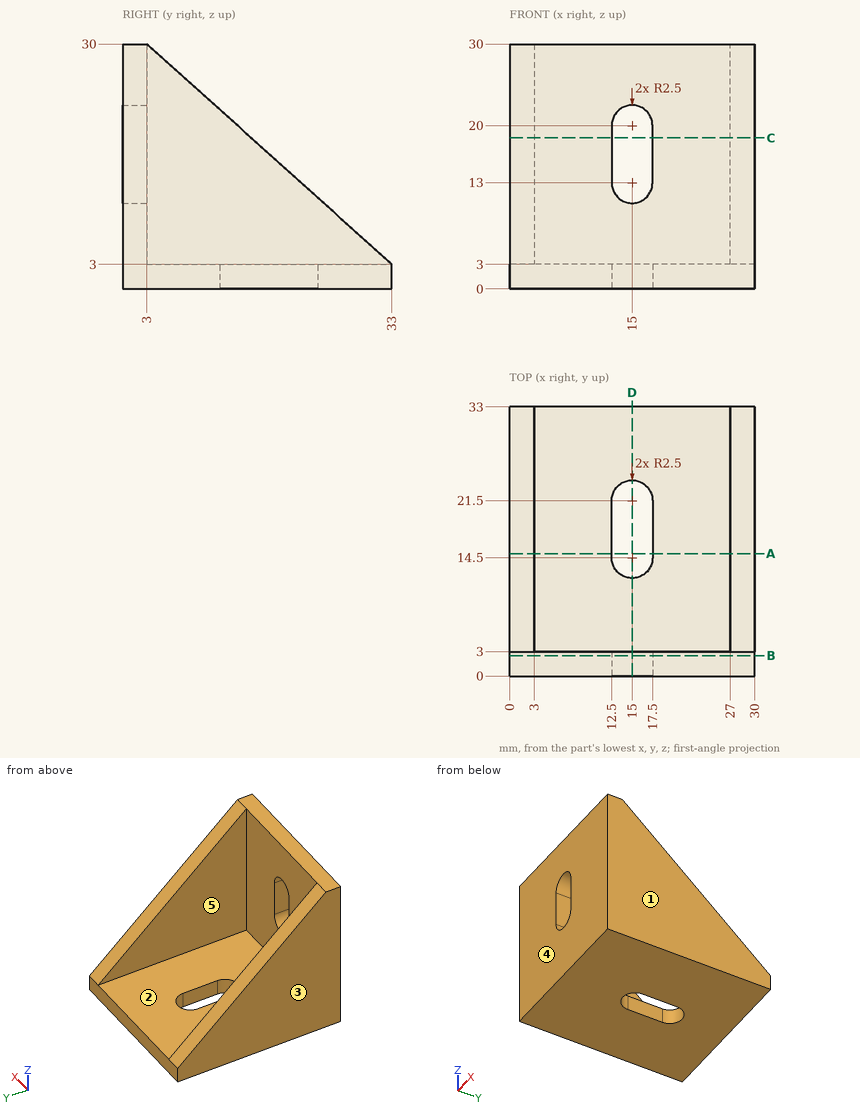
Answer from the drawing. Dimensions are ordinates in mm from the lowest x, y and z of the part. A direction names the side the tool comes from. Coordinates: 2 decimals unless noted, no trailing zeros. Write each loop counter-clockwise with the first axis right and the second up, starting at its lowest first coordinate (ties: lowest second). Pieces come first, ordered by that corner, then holes. Notation, with made-up numbers: (23.5, 44.25) - (58.5, 44.25) arc R17 ccw to (58.5, 75.25) - close; hole circle Ø2 at (72, -26.75). An arc over 180 degrees is marked (long way). Return JSON: item names as keys, results as strings. Group by question number.
Q1. The part is cut by section C-C on z = 18.5. Write down the section's boundary in (x, y).
Q2. The part is cut by section B-B on y = 2.5. Write down the section's boundary in (x, z), and give its area (3 significant figures).
Q3. The part is cut by section D-D on x = 15. Write down the section's boundary in (y, z).
Q4. Flat-ended cylindrical pins translate along their axes: pin 1 Ø1.5 at (x, y) = (22, 9.5) entering from +Z; pin 2 Ø8 at (x, z) = (8, 17.5) entering from +Y; pin 3 Ø6 at (x, y) = (25, 24) entering from +Z. Find the tip coordinate at first contact, or state that the pin passes through.
Q5. The part is cut by section A-A on y = 15. Write down the section's boundary in (x, z), and give its area (3 significant figures).
Q6. For a pull along X with two mould halves and no side action, classify the marked faces 3, 4 and 5 as +X half, -X half, draft (parallel to the pull), parting line (faces both ways), or undercut.
Q7. Which of the six approach directions +Z, -Z, +X, -X, +Y, -Y give full straight-line access (tool end or side, diameter ignored) to the marked faces 1 and 2?
Q8. Find the intervals of material crossed by line 1 along X through (y, z) = (12, 21.75); line 2 along X through (y, z) = (14.5, 1.25); line 3 along Y through (x, z) = (4, 23.25), in increasing order. Write a range as [from, to].
Evaluation:
{
 "1": {"outline": "(0, 0) - (12.5, 0) - (12.5, 3) - (3, 3) - (3, 15.78) - (0, 15.78) - close; (17.5, 0) - (30, 0) - (30, 15.78) - (27, 15.78) - (27, 3) - (17.5, 3) - close"},
 "2": {"outline": "(0, 0) - (30, 0) - (30, 30) - (0, 30) - close; hole (12.5, 13) arc R2.5 ccw to (17.5, 13) - (17.5, 20) arc R2.5 ccw to (12.5, 20) - close", "area": "845 mm2"},
 "3": {"outline": "(0, 0) - (12, 0) - (12, 3) - (3, 3) - (3, 10.5) - (0, 10.5) - close; (0, 22.5) - (3, 22.5) - (3, 30) - (0, 30) - close; (24, 0) - (33, 0) - (33, 3) - (24, 3) - close"},
 "4": {"pin 1": "stops at z = 3", "pin 2": "stops at y = 3", "pin 3": "stops at z = 13.11"},
 "5": {"outline": "(0, 0) - (12.5, 0) - (12.5, 3) - (3, 3) - (3, 19.2) - (0, 19.2) - close; (17.5, 0) - (30, 0) - (30, 19.2) - (27, 19.2) - (27, 3) - (17.5, 3) - close", "area": "172 mm2"},
 "6": {"face 3": "-X half", "face 4": "draft", "face 5": "undercut"},
 "7": {"face 1": "+Z, -Z, +X, +Y, -Y", "face 2": "+Z, +Y"},
 "8": {"line 1": "x = [0, 3], [27, 30]", "line 2": "x = [0, 12.5], [17.5, 30]", "line 3": "y = [0, 3]"}
}
